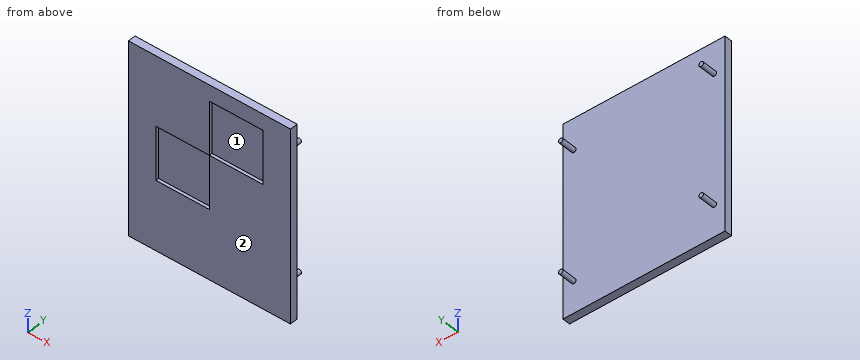
Autodesk Inventor part; units mm, degrees
ref_plane "YZ Plane" through (0, 0, 0) normal (1, 0, 0) x (0, 1, 0)
ref_plane "XZ Plane" through (0, 0, 0) normal (0, 1, 0) x (-1, 0, 0)
ref_plane "XY Plane" through (0, 0, 0) normal (0, 0, 1) x (1, 0, 0)
sketch "Boceto1" plane through (0, 0, 0) normal (0, 1, 0) x (-1, 0, 0)
  line L0 (53, 63) -> (-53, 63)
  line L1 (-53, 63) -> (-53, -63)
  line L2 (-53, -63) -> (53, -63)
  line L3 (53, -63) -> (53, 63)
  point P0 (0, 0)
  point P1 (0, 63)
  dimension "d1" = 106
  dimension "d2" = 126
  dimension "d3" = 53
  dimension "d4" = 63
extrude "Extrusión1" add sketch "Boceto1" along normal blind 5
sketch "Boceto2" plane through (0, 5, 0) normal (0, 1, 0) x (1, 0, 0)
  circle A0 centre (-45.929, -42.384) radius 1.5
  line L0 (-53, -63) -> (53, -63)
  line L1 (-53, 63) -> (-53, -63)
  line L2 (-81, 0) -> (77, 0)
  line L3 (0, -130) -> (0, 128)
  circle A1 centre (-45.929, 42.384) radius 1.5
  line L4 (-53, -63) -> (-53, 63)
  circle A2 centre (45.929, -42.384) radius 1.5
  circle A3 centre (45.929, 42.384) radius 1.5
  point P0 (0, 0)
  dimension "d7" = 3
  dimension "d8" = 20.616
  dimension "d9" = 7.071
extrude "Extrusión2" add sketch "Boceto2" along normal blind 10 contours A0 | A1 | A2 | A3
sketch "Boceto3" plane through (0, 0, 0) normal (0, -1, 0) x (1, 0, 0)
  line L0 (-35, 52.5) -> (35, 52.5)
  line L1 (35, 52.5) -> (35, -52.5)
  line L2 (35, -52.5) -> (-35, -52.5)
  line L3 (-35, -52.5) -> (-35, 52.5)
  line L4 (53, -63) -> (-53, -63)
  line L5 (-53, 63) -> (53, 63)
  line L6 (53, 63) -> (53, -63)
  line L7 (-53, -63) -> (-53, 63)
  line L8 (35, 17.5) -> (-35, 17.5)
  line L9 (35, -17.5) -> (-35, -17.5)
  line L10 (0, 52.5) -> (0, -52.5)
  point P0 (0, 0)
  point P1 (0, 17.5)
  point P2 (0, -17.5)
  dimension "d12" = 52.5
  dimension "d13" = 126
  dimension "d14" = 106
  dimension "d15" = 52.5
  dimension "d16" = 35
  dimension "d17" = 35
  dimension "d18" = 35
  dimension "d19" = 35
  dimension "d20" = 35
extrude "Extrusión3" cut sketch "Boceto3" against normal blind 2 contours L0 L1 L8 L10 | L8 L10 L9 L3
properties part number "Tapa 0"
Design review of the part built by this model. Coordinates are the model's own, in mm. Face numbers are marked on the shaded views. Round coordinates to 2 decimals unless told otherwise and drop trailing zeros. Write each loop counter-clockwise with the first axis right and the second up, starting at its lowest first coordinate (ties: lowest second). Pieces come first, ordered by that corner, then holes.
Item 1: Consider section D-D on x = 40. Give the boundary of the cut face in (y, z), and give its area (3 significant figures).
Item 2: Wall thickness on L1, parallel to Z at x = 21, y = 1.5; L2, parallel to Y at x = -20, z = -30; L3, parallel to Y at x = -16, z = 12: over which ranges is each line inside the solid? List them lowest first.
Item 3: Consider section C-C on y = 7.5. Give the boundary of the cut face in (x, z).
Item 4: For pin 1 Ø4 at (x, z) = (2.5, 16) entering from -Y; pin 2 Ø10 at (x, z) = (-27.5, -4.5) entering from -Y, all flat-tipped, find the tip position at first contact; note any pin that passes through.
Item 5: Consider section A-A on x = -8. Give the boundary of the cut face in (y, z).
Item 6: Consider section B-B on z = 39. Give the boundary of the cut face in (x, y), and give its area (3 significant figures).
Item 7: Draft analysis for pull direction Z (two halves, no side actions). For the marked faces 1 and 2, state which applies: released by +Z, released by -Z, zero draft, split by the parting line, or undercut.
Check values:
1. outline: (0, -63) - (5, -63) - (5, 63) - (0, 63) - close
1. area: 630 mm2
2. L1: z = -63 to 17.5, 52.5 to 63
2. L2: y = 0 to 5
2. L3: y = 2 to 5
3. outline: circle Ø3 at (-45.93, -42.38); circle Ø3 at (-45.93, 42.38); circle Ø3 at (45.93, -42.38); circle Ø3 at (45.93, 42.38)
4. pin 1: stops at y = 0
4. pin 2: stops at y = 2
5. outline: (0, -63) - (5, -63) - (5, 63) - (0, 63) - (0, 17.5) - (2, 17.5) - (2, -17.5) - (0, -17.5) - close
6. outline: (-53, 0) - (0, 0) - (0, 2) - (35, 2) - (35, 0) - (53, 0) - (53, 5) - (-53, 5) - close
6. area: 460 mm2
7. face 1: undercut
7. face 2: zero draft
